Verification items for the finished model (mm, model axes). A direction names the side the tool comes from. Coordinates: 2 decimals unless noted, no trailing zeros. Write each loop counter-clockwise with the first axis right and the second up, starting at its lowest first coordinate (ties: lowest second). Pieces come first, ordered by that corner, then holes. Notation, with made-up numbers: (-39.5, 45) - (-35.5, 45) arc R17 ccw to (-35.5, 75) - close; hole circle Ø4 at (2, 70). An arc over 180 degrees is marked (long way). Use one line per item in the form item = value. Start each with the question number.
(1) Sectioned sample at B-B (x = -90). Record the cut outline in (y, z), and give its area (3 significant figures).
(2) Mould release check, pull along Z, two halves, no side actions. Record for faces 1 (the flat face through (-49, 38.1, 0)), 2 (the flat face through (-49, -1, -25.4)), 3 (the cylindrical face through (-87.52, 37.11, 15.67)): released by +Z, released by -Z, zero draft, split by the parting line, or undercut.
(3) Sectioned sample at C-C (y = 18). Record the cut outline in (x, z).
(4) Sectioned sample at D-D (z = -8). Record the cut outline in (x, y).
(5) Tool access check on faces 4 (the flat face through (-49, -38.1, 0)), 5 (the flat face through (-49, 36.1, 0)), 6 (the cylindrical face through (-11.5, 37.1, 14)). Record the directions out of +Z, -Z, +X, -X, +Y, -Y that give a thin tool (end or side, any length) a straight path to the whole face; none if there is none.
(6) Material ranges on line 1 (X direction, y = 26.5, z = 24.15); line 2 (X direction, y = 37.1, z = 16); line 3 (Y direction, x = -50, z = 9), recorded low to high. Write a range as [from, to].
(7) Sectioned sample at A-A (z = 16). Record the cut outline in (x, y).
(8) Gauge pin test, flat end, axial feed: pin 1 Ø8 at (x, y) = (-70, -26.5) entering from +Z. Record the tip position at first contact, or that the pin passes through.
from build123d import *

# Parameters (mm, degrees)
SKETCH1_W             = 50.8
SKETCH1_H             = 76.2
BOSS_EXTRUDE1_DEPTH   = 100
SKETCH2_W             = 46.8
SKETCH2_H             = 72.2
CUT_EXTRUDE1_DEPTH    = 110.985317202
FILLET2_R             = 2
CORTAR_EXTRUIR2_DEPTH = 10
CROQUIS8_R            = 2.5
CORTAR_EXTRUIR8_DEPTH = 10


with BuildPart() as part:
    # Sketch1 → Boss-Extrude1 (new body)
    with BuildSketch(Plane(origin=(0, 0, 0), x_dir=(0, 0, -1), z_dir=(1, 0, 0))):
        Rectangle(SKETCH1_W, SKETCH1_H)
    extrude(amount=-BOSS_EXTRUDE1_DEPTH)

    # Sketch2 → Cut-Extrude1 (cut, through all)
    with BuildSketch(Plane(origin=(0, 0, 0), x_dir=(0, 0, -1), z_dir=(1, 0, 0))):
        Rectangle(SKETCH2_W, SKETCH2_H)
    extrude(amount=-CUT_EXTRUDE1_DEPTH, mode=Mode.SUBTRACT)

    # Fillet2
    fillet2_edges = [part.edges().sort_by_distance(p)[0] for p in [
        (-50, -36.1, 23.4),
        (-50, 36.1, 23.4),
        (-50, 36.1, -23.4),
        (-50, -36.1, -23.4),
        (-50, 38.1, 25.4),
        (-50, 38.1, -25.4),
        (-50, -38.1, -25.4),
        (-50, -38.1, 25.4),
    ]]
    fillet(fillet2_edges, radius=FILLET2_R)

    # Croquis2 → Cortar-Extruir2 (cut)
    with BuildSketch(Plane.XY.offset(25.4)):
        with BuildLine():
            ThreePointArc((-27, 26.5), (-30, 29.5), (-33, 26.5))
            Line((-33, 26.5), (-30, 26.5))
            Line((-30, 26.5), (-30, 23.5))
            ThreePointArc((-30, 23.5), (-27.878679656, 24.378679656), (-27, 26.5))
        make_face()
        with BuildLine():
            Line((-30, 26.5), (-33, 26.5))
            ThreePointArc((-33, 26.5), (-32.121320344, 24.378679656), (-30, 23.5))
            Line((-30, 23.5), (-30, 26.5))
        make_face()
        with BuildLine():
            ThreePointArc((-70, 23.5), (-67.878679656, 24.378679656), (-67, 26.5))
            Line((-67, 26.5), (-70, 26.5))
            Line((-70, 26.5), (-70, 23.5))
        make_face()
        with BuildLine():
            Line((-70, 26.5), (-67, 26.5))
            ThreePointArc((-67, 26.5), (-72.121320344, 28.621320344), (-70, 23.5))
            Line((-70, 23.5), (-70, 26.5))
        make_face()
        with BuildLine():
            ThreePointArc((-67, -26.5), (-67.878679656, -24.378679656), (-70, -23.5))
            Line((-70, -23.5), (-70, -26.5))
            Line((-70, -26.5), (-67, -26.5))
        make_face()
        with BuildLine():
            Line((-70, -26.5), (-70, -23.5))
            ThreePointArc((-70, -23.5), (-72.121320344, -28.621320344), (-67, -26.5))
            Line((-67, -26.5), (-70, -26.5))
        make_face()
        with BuildLine():
            ThreePointArc((-27, -26.5), (-27.878679656, -24.378679656), (-30, -23.5))
            Line((-30, -23.5), (-30, -26.5))
            Line((-30, -26.5), (-33, -26.5))
            ThreePointArc((-33, -26.5), (-30, -29.5), (-27, -26.5))
        make_face()
        with BuildLine():
            Line((-30, -26.5), (-30, -23.5))
            ThreePointArc((-30, -23.5), (-32.121320344, -24.378679656), (-33, -26.5))
            Line((-33, -26.5), (-30, -26.5))
        make_face()
    extrude(amount=-CORTAR_EXTRUIR2_DEPTH, mode=Mode.SUBTRACT)

    # Croquis8 → Cortar-Extruir8 (cut)
    with BuildSketch(Plane(origin=(0, 38.1, 0), x_dir=(1, 0, 0), z_dir=(0, 1, 0))):
        with Locations(Location((-90, 16, 0), (0, 0, 270))):
            Circle(CROQUIS8_R)
        with Locations(Location((-10, 16, 0), (0, 0, 270))):
            Circle(CROQUIS8_R)
        with Locations(Location((-90, -16, 0), (0, 0, 270))):
            Circle(CROQUIS8_R)
        with Locations(Location((-10, -16, 0), (0, 0, 270))):
            Circle(CROQUIS8_R)
    extrude(amount=-CORTAR_EXTRUIR8_DEPTH, mode=Mode.SUBTRACT)


solid = part.part
Answers below:
q1.outline = (-38.1, -23.4) arc R2 ccw to (-36.1, -25.4) - (36.1, -25.4) arc R2 ccw to (38.1, -23.4) - (38.1, -18.5) - (36.1, -18.5) - (36.1, -21.4) arc R2 cw to (34.1, -23.4) - (-34.1, -23.4) arc R2 cw to (-36.1, -21.4) - (-36.1, 21.4) arc R2 cw to (-34.1, 23.4) - (34.1, 23.4) arc R2 cw to (36.1, 21.4) - (36.1, 18.5) - (38.1, 18.5) - (38.1, 23.4) arc R2 ccw to (36.1, 25.4) - (-36.1, 25.4) arc R2 ccw to (-38.1, 23.4) - close; (36.1, -13.5) - (38.1, -13.5) - (38.1, 13.5) - (36.1, 13.5) - close
q1.area = 472 mm2
q2.face_1 = zero draft
q2.face_2 = released by -Z
q2.face_3 = undercut
q3.outline = (-100, -25.4) - (0, -25.4) - (0, -23.4) - (-100, -23.4) - close; (-100, 23.4) - (0, 23.4) - (0, 25.4) - (-100, 25.4) - close
q4.outline = (-100, -38.1) - (0, -38.1) - (0, -36.1) - (-100, -36.1) - close; (-100, 36.1) - (0, 36.1) - (0, 38.1) - (-100, 38.1) - close
q5.face_4 = +Z, -Z, +X, -X, -Y
q5.face_5 = +X, -X
q5.face_6 = +Y
q6.line_1 = [-100, -73], [-67, -33], [-27, 0]
q6.line_2 = [-100, -92.5], [-87.5, -12.5], [-7.5, 0]
q6.line_3 = [-38.1, -36.1], [36.1, 38.1]
q7.outline = (-100, -38.1) - (0, -38.1) - (0, -36.1) - (-100, -36.1) - close; (-100, 36.1) - (-92.5, 36.1) - (-92.5, 38.1) - (-100, 38.1) - close; (-87.5, 36.1) - (-12.5, 36.1) - (-12.5, 38.1) - (-87.5, 38.1) - close; (-7.5, 36.1) - (0, 36.1) - (0, 38.1) - (-7.5, 38.1) - close
q8.pin_1 = 25.4
